Geometry: final body of the model. Coordinates: model frame, mm. Coordinates: 2 decimals unless noted, no trailing zeros. Write each loop counter-clockwise with the first axis right and the second up, starting at its lowest first coordinate (ties: lowest second). Pieces come first, ordered by that corner, then holes. Notation, with made-up numbers: (35.25, 84.5) - (45.25, 84.5) arc R18 ccw to (45.25, 89.5) - close; hole circle Ø1 at (7.5, 46.5). An arc over 180 degrees is marked (long way). Answer as a JSON object with one key per item and string values. Group by question number.
Item 1: Line query: line 1 along Y through (x, z) = (0, -1.5); line 2 along X through (y, z) = (0, 0.5); line 3 along X through (y, z) = (-0.1, 2.25). Output: solid intervals per line, ascending. Write a range as from..to.
Item 2: First-contact query: pin 1 Ø0.9 at (x, y) = (1, 0.5) entering from +Z; pin 2 Ø2 at (x, y) = (1.5, -1.5) entering from +Z; pin 3 Ø1 at (y, z) = (-1, -1) entering from +X. Flat tips, straight axial feed; report the tip coordinate or a pass-through.
Item 3: Mould query, pull axis X, two halves, no side actions, for faces 1 (the conical face through (-1.08, -0.77, 2.42)), 2 (the flat face through (1, -1, -4.35)), 3 (the cylindrical face through (1.42, 0.48, 0.86)), 4 (the cylindrical face through (1, 0, -1)). Classes: pulls with the +X half, pulls with the -X half, needs draft (parallel to the pull), parting line crosses it, or undercut.
Item 4: Section B-B on x = -0.25. Return loops of the section in (y, z).
Item 5: Section C-C on z = -2. Return loops of the section in (x, y), and give its area (3 significant figures).
Item 6: Section D-D on z = 1. Return loops of the section in (x, y), and give its area (3 significant figures).
```python
from build123d import *

# Parameters (mm, degrees)
F0_R      = 1.5
F0_R_2    = 1
F1_DEPTH  = 2.6
F5_COUNT  = 5
F5_ANGLE  = 288
F17_DEPTH = 1.64
F0_R_3    = 1.9
F18_DEPTH = 4.35


with BuildPart() as f1:
    # F0 (on Top) → F1 (new body)
    with BuildSketch(Plane.XY):
        Circle(F0_R)
        Circle(F0_R_2, mode=Mode.SUBTRACT)
    extrude(amount=F1_DEPTH)


with BuildPart() as f4:
    # F3 (on Front) → F4 (revolve)
    with BuildSketch(Plane.XZ):
        Polygon((0.9303738137, 2.820600407), (1.375, 1.599), (1.9388155725, 1.804212086), align=None)
    revolve(axis=Axis((1.1526869068, 0, 2.2098002035), (-0.3420201433, 0, 0.9396926208)))


with BuildPart() as f5_1:
    # F5: instance of F4
    add(f4.part.rotate(Axis((0, 0, 0.7995), (0, 0, 1)), 1 * F5_ANGLE / (F5_COUNT - 1)))


with BuildPart() as f5_2:
    # F5: instance of F4
    add(f4.part.rotate(Axis((0, 0, 0.7995), (0, 0, 1)), 2 * F5_ANGLE / (F5_COUNT - 1)))


with BuildPart() as f5_3:
    # F5: instance of F4
    add(f4.part.rotate(Axis((0, 0, 0.7995), (0, 0, 1)), 3 * F5_ANGLE / (F5_COUNT - 1)))


with BuildPart() as f5_4:
    # F5: instance of F4
    add(f4.part.rotate(Axis((0, 0, 0.7995), (0, 0, 1)), 4 * F5_ANGLE / (F5_COUNT - 1)))


with BuildPart() as f6_1:
    # F6: copy of F1
    add(f1.part)


with BuildPart() as f1_1:
    add(f1.part)

    # F7: intersect F4
    add(f4.part, mode=Mode.INTERSECT)



with BuildPart() as f8_1:
    # F8: copy of F6_1
    add(f6_1.part)


with BuildPart() as f9_1:
    # F9: copy of F8_1
    add(f8_1.part)


with BuildPart() as f10_1:
    # F10: copy of F9_1
    add(f9_1.part)


with BuildPart() as f5_1_1:
    add(f5_1.part)

    # F11: intersect F6_1
    add(f6_1.part, mode=Mode.INTERSECT)


with BuildPart() as f5_2_1:
    add(f5_2.part)

    # F12: intersect F8_1
    add(f8_1.part, mode=Mode.INTERSECT)


with BuildPart() as f5_3_1:
    add(f5_3.part)

    # F13: intersect F9_1
    add(f9_1.part, mode=Mode.INTERSECT)


with BuildPart() as f14_1:
    # F14: copy of F10_1
    add(f10_1.part)


with BuildPart() as f10_1_1:
    add(f10_1.part)

    # F15: intersect F5_4
    add(f5_4.part, mode=Mode.INTERSECT)


with BuildPart() as f17:
    # F0 (on Top) → F17 (new body)
    with BuildSketch(Plane.XY):
        Circle(F0_R)
        Circle(F0_R_2, mode=Mode.SUBTRACT)
    extrude(amount=F17_DEPTH)


with BuildPart() as f1_2:
    add(f1_1.part)

    add(f5_1_1.part)  # F18 merges F5_1

    add(f5_2_1.part)  # F18 merges F5_2

    add(f5_3_1.part)  # F18 merges F5_3

    add(f10_1_1.part)  # F18 merges F10_1

    add(f17.part)  # F18 merges F17
    # F0 (on Top) → F18 (join)
    with BuildSketch(Plane.XY):
        Circle(F0_R_3)
        Circle(F0_R, mode=Mode.SUBTRACT)
        Circle(F0_R)
        Circle(F0_R_2, mode=Mode.SUBTRACT)
    extrude(amount=-F18_DEPTH)


solid = f1_2.part
```
Checks:
{
 "1": {"line 1": "-1.9..-1, 1..1.9", "line 2": "-1.5..-1, 1..1.5", "line 3": "0.99..1.48"},
 "2": {"pin 1": "z = 2.6", "pin 2": "z = 2.38", "pin 3": "x = 1.83"},
 "3": {"face 1": "undercut", "face 2": "needs draft", "face 3": "parting line crosses it", "face 4": "undercut"},
 "4": {"outline": "(-1.88, -4.35) - (-0.97, -4.35) - (-0.97, 1.64) - (-1.48, 1.64) - (-1.48, 0) - (-1.88, 0) - close; (0.97, -4.35) - (1.88, -4.35) - (1.88, 0) - (1.48, 0) - (1.48, 1.64) - (0.97, 1.64) - close"},
 "5": {"outline": "circle Ø3.8 at (0, 0); hole circle Ø2 at (0, 0)", "area": "8.20 mm^2"},
 "6": {"outline": "circle Ø3 at (0, 0); hole circle Ø2 at (0, 0)", "area": "3.93 mm^2"}
}
